The listing builds one solid part. Answer for the finished solid, in the listing's coordinates (mm). Face numbers are marked on the shaded views. A direction names the side the tool comes from. Round coordinates to 2 decimals unless told otherwise and drop trailing zeros. Loops run counter-clockwise (first coordinate to the right, second up) from the corner with the lowest first, then second, coordinate; pieces in that order, holes last. Notation, with made-up numbers: (-3, -14.5) -> (46, -14.5) arc R24 ccw to (46, 13.5) -> close; hole circle Ø4 at (-37.5, -5). An arc over 180 degrees is marked (long way). Write each question's results on one line, items separated by ' | '. Start each with the question number.
(1) The part is cut by section C-C (y = 12.5). Determine the outline of the cut face in (x, z), plus the area to 3 significant figures.
(2) The part is cut by section A-A (x = 60). Determine the outline of the cut face in (y, z).
(3) Flat-ended cylindrical pins translate along their axes: pin 1 (4.5 mm diameter, centred on x = -22, z = -73, fed in from +Y); pin 2 (3 mm diameter, centred on x = -31.5, y = 18, fed in from +Z); pin 3 (1.5 mm diameter, centred on x = -36.5, y = 13.5, fed in from -Z). Find the tip coordinate at first contact, or state that the pin passes through.
(4) For the marked faces 1 and 2, determine the directions among +Z, -Z, +X, -X, +Y, -Y from which every point of the face is accessible in a straight line to the end or side of a thin tool.
(5) Straight lines are drawn through the part: probe 1 along Z at (x, y) = (-38.5, 13); probe 2 along Y at (x, z) = (42.5, 75.5). For each, find the intervals that lie inside material, in ascending order.
(6) The part is cut by section B-B (z = -72). Determine the outline of the cut face in (x, y), plus the area to 3 significant figures.
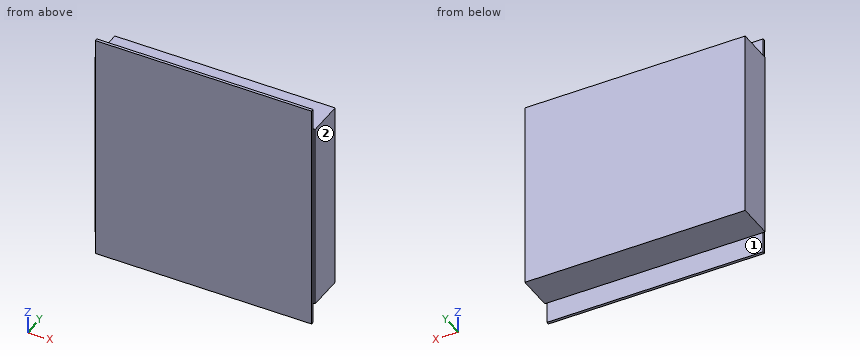
```python
from build123d import *

# Parameters (mm, degrees)
SKETCH_1_W      = 158
SKETCH_1_H      = 136
EXTRUDE_1_DEPTH = 26
SKETCH_2_W      = 155
SKETCH_2_H      = 166
EXTRUDE_2_DEPTH = 2


with BuildPart() as part:
    # 草图1 → 拉伸1 (new body)
    with BuildSketch(Plane(origin=(0, 0, 0), x_dir=(1, 0, 0), z_dir=(0, 1, 0))):
        Rectangle(SKETCH_1_W, SKETCH_1_H)
    extrude(amount=EXTRUDE_1_DEPTH)

    # 草图2 → 拉伸2 (add)
    with BuildSketch(Plane.XZ):
        Rectangle(SKETCH_2_W, SKETCH_2_H)
    extrude(amount=EXTRUDE_2_DEPTH)


solid = part.part
```
Checked values:
1) outline: (-79, -68) -> (79, -68) -> (79, 68) -> (-79, 68) -> close | area: 21,500 mm2
2) outline: (-2, -83) -> (0, -83) -> (0, -68) -> (26, -68) -> (26, 68) -> (0, 68) -> (0, 83) -> (-2, 83) -> close
3) pin 1: stops at y = 0 | pin 2: stops at z = 68 | pin 3: stops at z = -68
4) face 1: -Z, +X, -X, +Y | face 2: +Z, -Z, +X, +Y, -Y
5) probe 1: z = -68 to 68 | probe 2: y = -2 to 0
6) outline: (-77.5, -2) -> (77.5, -2) -> (77.5, 0) -> (-77.5, 0) -> close | area: 310 mm2
